from build123d import *

# Parameters (mm, degrees)
F0_W     = 762
F0_H     = 381
F0_W_2   = 660.4
F0_H_2   = 279.4
F1_DEPTH = 381
F2_W     = 381
F2_H     = 177.8
F3_DEPTH = 1270
F4_R     = 38.1
F5_DEPTH = 1270


with BuildPart() as f1:
    # F0 (on Top) → F1 (new body)
    with BuildSketch(Plane.XY):
        Rectangle(F0_W, F0_H)
        Rectangle(F0_W_2, F0_H_2, mode=Mode.SUBTRACT)
    extrude(amount=F1_DEPTH)

    # F2 (on face) → F3 (cut)
    with BuildSketch(Plane.XZ.offset(190.5)):
        with Locations((0, 292.1)):
            Rectangle(F2_W, F2_H)
    extrude(amount=-F3_DEPTH, mode=Mode.SUBTRACT)

    # F4 (on face) → F5 (cut)
    with BuildSketch(Plane.YZ.offset(381)):
        with Locations((0, 190.5)):
            Circle(F4_R)
    extrude(amount=-F5_DEPTH, mode=Mode.SUBTRACT)


solid = f1.part
Design review of the part built by this model. Coordinates are the model's own, in mm. A direction names the side the tool comes from. Coordinates: 2 decimals unless noted, no trailing zeros. Loops run counter-clockwise (first coordinate to the right, second up) from the corner with the lowest first, then second, coordinate; pieces in that order, holes last. Notation, with made-up numbers: (24.25, 37) - (64.25, 37) arc R17 cw to (64.25, 66) - close; hole circle Ø10 at (69.25, 1.5). An arc over 180 degrees is marked (long way). Use CSV: the item, a comma, the result in double quotes. Start each with the question number.
1. Add section C-C on x = 183. Give the boundary of the cut face in (y, z), plus the area to 3 significant figures.
2. Add section A-A on y = 0. Give the boundary of the cut face in (x, z), plus the area to 3 significant figures.
3. To check wall thickness, follow probe 1 along X at (y, z) = (-94, 360.5); probe 2 along Z at (x, y) = (359.5, 0); probe 3 along Y at (x, z) = (-283, 295). State the ranges of each line that lie inside material, in increasing order.
4. Mouldability with a two-part tool opening along Z and no side actions: class faces 1 (the flat face through (-3, 165, 203.2)), 2 (the cylindrical face through (355.956, -8.259, 153.306)), 3 (the flat face through (381, 40, 188)), 4 (the cylindrical face through (-355.244, -8.259, 153.306)) as released by +Z, released by -Z, zero draft, split by the parting line, or undercut.
5. For faces 5 (the flat face through (-190.5, -165, 291)), 6 (the flat face through (-5, -139.7, 145)), 7 (the flat face through (348, 3, 381)), list the 3-axis set-ups (+Z, -Z, +X, -X, +Y, -Y) from which the entire face can be reached by the end or side of a thin tool; tool diameter is ignored.
6. Add section B-B on z = 190.5. Give the boundary of the cut face in (x, y).
7. Add section D-D on z = 102.5. Give the boundary of the cut face in (x, y), plus the area to 3 significant figures.
Resolved:
1,outline,"(-190.5, 0) - (-139.7, 0) - (-139.7, 203.2) - (-190.5, 203.2) - close; (139.7, 0) - (190.5, 0) - (190.5, 203.2) - (139.7, 203.2) - close"
1,area,"20,600 mm2"
2,outline,"(-381, 0) - (-330.2, 0) - (-330.2, 152.4) - (-381, 152.4) - close; (-381, 228.6) - (-330.2, 228.6) - (-330.2, 381) - (-381, 381) - close; (330.2, 0) - (381, 0) - (381, 152.4) - (330.2, 152.4) - close; (330.2, 228.6) - (381, 228.6) - (381, 381) - (330.2, 381) - close"
2,area,"31,000 mm2"
3,probe 1,"-381 to -330.2, 330.2 to 381"
3,probe 2,"0 to 152.4, 228.6 to 381"
3,probe 3,"-190.5 to -139.7, 139.7 to 190.5"
4,face 1,"released by +Z"
4,face 2,"undercut"
4,face 3,"zero draft"
4,face 4,"undercut"
5,face 5,"+Z, +Y, -Y"
5,face 6,"+Z, -Z"
5,face 7,"+Z, +X, -X, +Y, -Y"
6,outline,"(-381, -190.5) - (381, -190.5) - (381, -38.1) - (330.2, -38.1) - (330.2, -139.7) - (-330.2, -139.7) - (-330.2, -38.1) - (-381, -38.1) - close; (-381, 38.1) - (-330.2, 38.1) - (-330.2, 139.7) - (330.2, 139.7) - (330.2, 38.1) - (381, 38.1) - (381, 190.5) - (-381, 190.5) - close"
7,outline,"(-381, -190.5) - (381, -190.5) - (381, 190.5) - (-381, 190.5) - close; hole (-330.2, -139.7) - (330.2, -139.7) - (330.2, 139.7) - (-330.2, 139.7) - close"
7,area,"106,000 mm2"
